from build123d import *

# Parameters (mm, degrees)
F1_DEPTH = 30


with BuildPart() as f1:
    # F0 (on Front) → F1 (new body)
    with BuildSketch(Plane.XZ):
        with BuildLine():
            Line((-103.501727, 24.947246), (-103.501727, -45.052754))
            Line((-103.501727, -45.052754), (-73.501727, -45.052754))
            Line((-73.501727, -45.052754), (-73.501727, -25.052754))
            ThreePointArc((-73.501727, -25.052754), (-70.572794, -17.981686), (-63.501727, -15.052754))
            Line((-63.501727, -15.052754), (-60.501727, -15.052754))
            ThreePointArc((-60.501727, -15.052754), (-53.430659, -17.981686), (-50.501727, -25.052754))
            Line((-50.501727, -25.052754), (-50.501727, -45.052754))
            Line((-50.501727, -45.052754), (9.498273, -45.052754))
            Line((9.498273, -45.052754), (9.498273, -25.052754))
            ThreePointArc((9.498273, -25.052754), (12.427206, -17.981686), (19.498273, -15.052754))
            Line((19.498273, -15.052754), (22.498273, -15.052754))
            ThreePointArc((22.498273, -15.052754), (29.569341, -17.981686), (32.498273, -25.052754))
            Line((32.498273, -25.052754), (32.498273, -45.052754))
            Line((32.498273, -45.052754), (72.498273, -45.052754))
            Line((72.498273, -45.052754), (72.498273, -1.052754))
            Line((72.498273, -1.052754), (31.498273, 44.947246))
            Line((31.498273, 44.947246), (-3.501727, 44.947246))
            Line((-3.501727, 44.947246), (-3.501727, 19.947246))
            ThreePointArc((-3.501727, 19.947246), (-7.895125, 9.340645), (-18.501727, 4.947246))
            ThreePointArc((-18.501727, 4.947246), (-29.108328, 9.340645), (-33.501727, 19.947246))
            Line((-33.501727, 19.947246), (-33.501727, 44.947246))
            Line((-33.501727, 44.947246), (-83.501727, 44.947246))
            ThreePointArc((-83.501727, 44.947246), (-97.643862, 39.089382), (-103.501727, 24.947246))
        make_face()
    extrude(amount=F1_DEPTH)


solid = f1.part
Here's how the part is built. I have some questions about the finished solid (model axes, mm). A direction names the side the tool comes from. Give positions to 0.01 mm unless a question says otherwise; leave off trailing zeros. Order: outer loops, then holes, each group sorted by start corner. A loop starts at its lowest first (then second) coordinate and runs counter-clockwise, first axis right, second up. Notation, with made-up numbers: M -7.5,67 L 49.5,67 A35 ccw 49.5,100 Z; hole C -18,85.5 d4. An arc over 180 degrees is marked long. Answer as a JSON object with one key per item and string values. Group by question number.
1) Suppose I cut it at D-D, the plane x = -65.5. Write out the boundary of the cut face in (y, z), plus the area to 3 significant figures.
2) Suppose I cut it at C-C, the plane y = -17. Write out the boundary of the cut face in (x, z).
3) I'm going to push flat-ended pins straight in: pin 1 Ø0.9 at (x, y) = (-62, -16) entering from -Z; pin 2 Ø1.5 at (y, z) = (-24, 35.5) entering from -X; pin 3 Ø1.5 at (x, y) = (53, -19.5) entering from +Z; pin 4 Ø1.5 at (x, z) = (-70, 27.5) entering from +Y. Where does each tip first touch, or does it pass through?
4) Please list where these lines run through material, in increasing order: L1, parallel to X at y = -15, z = -39; L2, parallel to Z at x = -63.5, y = -19.25; L3, parallel to X at y = -4, z = 7. Write a range as [from, to].
5) Suppose I cut it at A-A, the plane z = -37.5. Write out the boundary of the cut face in (x, y).
6) Suppose I cut it at B-B, the plane z = 34.5. Write out the boundary of the cut face in (x, y), plus the area to 3 significant figures.
7) We'd pull the mould along X, two halves only. Please class faces 1 (the flat face through (52.285, -14.79, 21.625)), 2 (the cylindrical face through (-97.49, -14.79, 39.24)), 3 (the flat face through (-33.502, -15, 32)), 4 (the flat face through (-17, 0, 1)): pulls with the +X half, pulls with the -X half, needs draft (parallel to the pull), parting line crosses it, or undercut.
8) On a 3-axis mill with a long thin cutter (end or side, diameter ignored), from which of +Z, -Z, +X, -X, +Y, -Y can I reach the whole of each face in a straight line? I mean faces 5 (the flat face through (-3.502, -15, 33)), 6 (the cylindrical face through (-70.65, -14.79, -18.06)), 7 (the flat face through (14, -15, 44.947)). Say none if no direction works.
Results found:
{
 "1": {"outline": "M -30,-15.25 L 0,-15.25 L 0,44.95 L -30,44.95 Z", "area": "1,810 mm²"},
 "2": {"outline": "M -103.5,-45.05 L -73.5,-45.05 L -73.5,-25.05 A10 cw -63.5,-15.05 L -60.5,-15.05 A10 cw -50.5,-25.05 L -50.5,-45.05 L 9.5,-45.05 L 9.5,-25.05 A10 cw 19.5,-15.05 L 22.5,-15.05 A10 cw 32.5,-25.05 L 32.5,-45.05 L 72.5,-45.05 L 72.5,-1.05 L 31.5,44.95 L -3.5,44.95 L -3.5,19.95 A15 cw -18.5,4.95 A15 cw -33.5,19.95 L -33.5,44.95 L -83.5,44.95 A20 ccw -103.5,24.95 Z"},
 "3": {"pin 1": "z = -15.05", "pin 2": "x = -100.93", "pin 3": "z = 21.66", "pin 4": "y = 0"},
 "4": {"L1": "[-103.5, -73.5], [-50.5, 9.5], [32.5, 72.5]", "L2": "[-15.05, 44.95]", "L3": "[-103.5, -26.08], [-10.93, 65.32]"},
 "5": {"outline": "M -103.5,-30 L -73.5,-30 L -73.5,0 L -103.5,0 Z; M -50.5,-30 L 9.5,-30 L 9.5,0 L -50.5,0 Z; M 32.5,-30 L 72.5,-30 L 72.5,0 L 32.5,0 Z"},
 "6": {"outline": "M -101.07,-30 L -33.5,-30 L -33.5,0 L -101.07,0 Z; M -3.5,-30 L 40.81,-30 L 40.81,0 L -3.5,0 Z", "area": "3,360 mm²"},
 "7": {"face 1": "pulls with the +X half", "face 2": "pulls with the -X half", "face 3": "undercut", "face 4": "needs draft"},
 "8": {"face 5": "+Z, +Y, -Y", "face 6": "-Z, +Y, -Y", "face 7": "+Z, +X, -X, +Y, -Y"}
}
